```python
from build123d import *

# Parameters (mm, degrees)
FILLET1_R          = 1
SKETCH2_R          = 0.75
CUT_EXTRUDE1_DEPTH = 9
CIRPATTERN1_COUNT  = 16
SKETCH3_R          = 0.5
CUT_EXTRUDE2_DEPTH = 9.0000001


with BuildPart() as part:
    # Sketch1 → Revolve1 (revolve)
    with BuildSketch(Plane.XY):
        Polygon((-2.765, 0), (-2.765, 2.891054023), (0, 2.891054023), (0, 8), (-6, 8), (-6, 1.24483654), (-4.003398957, 1.24483654), (-3.067620744, 0), align=None)
    revolve(axis=Axis((0, 2.891054023, 0), (0, 1, 0)))

    # Fillet1
    fillet1_edges = [part.edges().sort_by_distance(p)[0] for p in [
        (6, 8, 0),
    ]]
    fillet(fillet1_edges, radius=FILLET1_R)

    # Sketch2 → Cut-Extrude1 (cut, through all)
    with BuildSketch(Plane(origin=(0, 0, 0), x_dir=(1, 0, 0), z_dir=(0, 1, 0))):
        with Locations((0, 6.5)):
            Circle(SKETCH2_R)
    cut_extrude1 = extrude(amount=CUT_EXTRUDE1_DEPTH, mode=Mode.SUBTRACT)

    # CirPattern1: Cut-Extrude1 ×16 about axis
    cirpattern1_axis = Axis((0, 0, 0), (0, 1, 0))
    for i in range(1, CIRPATTERN1_COUNT):
        add(cut_extrude1.rotate(cirpattern1_axis, i * 360 / CIRPATTERN1_COUNT), mode=Mode.SUBTRACT)

    # Sketch3 → Cut-Extrude2 (cut, through all)
    with BuildSketch(Plane(origin=(0, 0, 0), x_dir=(1, 0, 0), z_dir=(0, 1, 0))):
        Circle(SKETCH3_R)
    extrude(amount=CUT_EXTRUDE2_DEPTH, mode=Mode.SUBTRACT)


solid = part.part
```
Can you work these out from the model? Positions are in its coordinate system, mm. Coordinates: 2 decimals unless noted, no trailing zeros. Loops run counter-clockwise (first coordinate to the right, second up) from the corner with the lowest first, then second, coordinate; pieces in that order, holes last. Notation, with made-up numbers: (83.5, 7.5) -> (111.5, 7.5) arc R15 cw to (111.5, 13.5) -> close; hole circle Ø6 at (51.5, 73.25). An arc over 180 degrees is marked (long way). Put each result on its own line as item: value. Start each with the question number.
Q1. Thinking about a two-plate mould opening in Z: for faces 1 (the face through (-5.31, 4.41, 2.21)), 2 (the face through (-5.75, 4.41, 0.01)), 3 (the face through (4.99, 4.08, -3.33)), 4 (the face through (4.984, 4.082, 3.341)), which applies, pulls with the +Z half, pulls with the -Z half, needs draft (parallel to the pull), parting line crosses it, or undercut?
Q2. If I drill on line 1 (Z direction, x = 0, y = 1.9) (3 decimals); line 2 (Y direction, x = 0.25, z = 2.5); line 3 (Y direction, x = 5, z = 0.75), over which ranges is the centre line in solid material (lowest first)? Write a range as [from, to].
Q3. I'm going to push flat-ended pins straight in: P1, Ø3.5, axis at x = 0, z = 0, coming from the -Y side; P2, Ø2, axis at y = 4.5, z = 2.5, coming from the +X side; P3, Ø1, axis at x = 0, z = -4, coming from the -Y side. Where does each tip first touch, or does it pass through?
Q4. I want a section at A-A (x = 0). Write out the boundary of the cut face in (y, z) (3 decimals), plus the area to 3 significant figures.
Taken from the geometry:
1. face 1: undercut
1. face 2: undercut
1. face 3: pulls with the -Z half
1. face 4: pulls with the +Z half
2. line 1: z = [-5.75, -2.765], [2.765, 5.75]
2. line 2: y = [2.89, 8]
2. line 3: y = [1.24, 8]
3. P1: stops at y = 2.89
3. P2: stops at x = 5.81
3. P3: stops at y = 0.58
4. outline: (0, -3.068) -> (1.245, -4.003) -> (1.245, -5.75) -> (7.661, -5.75) arc R1 ccw to (8, -5) -> (8, -0.5) -> (2.891, -0.5) -> (2.891, -2.765) -> (0, -2.765) -> close; (0, 2.765) -> (2.891, 2.765) -> (2.891, 0.5) -> (8, 0.5) -> (8, 5) arc R1 ccw to (7.661, 5.75) -> (1.245, 5.75) -> (1.245, 4.003) -> (0, 3.068) -> close
4. area: 65.2 mm2
